Part model, mm, in its own coordinate system. A direction names the side the tool comes from. Round coordinates to 2 decimals unless told otherwise and drop trailing zeros. Order: outer loops, then holes, each group sorted by start corner. A loop starts at its lowest first (then second) coordinate and runs counter-clockwise, first axis right, second up. Notation, with made-up numbers: M 21,71 L 34,71 A14 cw 34,77 Z; hole C -26,39 d4. An arc over 180 degrees is marked long. Write each question's results on one line, items separated by ' | '. Start each with the question number.
1. Band-saw the part on C-C, the plane x = 40. List the corners of the cut face in (y, z).
2. Two-plate mould, pull along X, no slides. Class faces 3 (the face through (69.89, -30.02, 7.46)), 4 (the face through (41.068, -25.451, 7.465)), 5 (the face through (84.52, -17.57, 7.46)): +X half, -X half, draft (parallel to the pull), parting line (faces both ways), or undercut.
3. Band-saw the part on D-D, the plane z = 8.45. Give the number of separate pieces and of enclosed holes in the cut face, then the cut area to 3 significant figures.
4. Probe L1, parallel to Y at x = 60, z = 5.9; L2, parallel to Y at x = 49.5, z = 8.9; L3, parallel to X at y = -24.5, z = 7.8. List the from-to ranges inside material, lowest first. Write a range as [from, to].
5. Drop flat-ended pins along their axis: pin 1 Ø3.5 at (x, y) = (59.85, -25.73) entering from -Z; pin 2 Ø2 at (y, z) = (-3.5, 9) entering from -X; pin 3 Ø1 at (y, z) = (-14, 9.5) entering from -X. Give the stop position or say it passes through.
6. Band-saw the part on B-B, the plane x = 62.5. List the corners of the cut face in (y, z), then the cut area to 3 significant figures.
7. Which spindle directions (+Z, -Z, +X, -X, +Y, -Y) get a long thin tool onto all of the face, cutting with end or side? Do faces 1 (the face through (45, 0, 7)), 2 (the face through (93.45, -26.96, 7.54)). Say none if no direction does.
8. Band-saw the part on A-A, the plane y = 0. List the corners of the cut face in (x, z), then the cut area to 3 significant figures.
```python
from build123d import *

# Parameters (mm, degrees)
EXTRUDE_1_DEPTH     = 15
FILLET_1_R          = 5
FILLET_2_R          = 5
FILLET_3_R          = 5
FILLET_4_R          = 5
FILLET_5_R          = 5
FILLET_6_R          = 5
FILLET_7_R          = 5
FILLET_8_R          = 5
FILLET_9_R          = 5
FILLET_10_R         = 5
FILLET_11_R         = 5
FILLET_12_R         = 5
FILLET_13_R         = 5
FILLET_14_R         = 5
FILLET_15_R         = 5
FILLET_16_R         = 5
SKETCH_5_R          = 1.5
CUT_EXTRUDE_1_DEPTH = 15
CUT_EXTRUDE_START   = -15
SKETCH_6_R          = 1.5
CUT_EXTRUDE_5_DEPTH = 15
EXTRUDE_2_DEPTH     = 15
FILLET_17_R         = 5
FILLET_18_R         = 5
FILLET_19_R         = 5
FILLET_20_R         = 5
SKETCH_8_W          = 96.520141499
SKETCH_8_H          = 72.316132992
CUT_EXTRUDE_6_DEPTH = 5
SKETCH_9_W          = 91.216327174
SKETCH_9_H          = 79.967676963
CUT_EXTRUDE_7_DEPTH = 5


with BuildPart() as part:
    # 草图3 → 凸台-拉伸1 (new body)
    with BuildSketch(Plane.XY):
        with BuildLine():
            Line((101.99145665, -27.727634828), (114.18506552, -15.283623844))
            ThreePointArc((114.18506552, -15.283623844), (110, 0), (114.18506552, 15.283623844))
            Line((114.18506552, 15.283623844), (101.99145665, 27.727634828))
            Line((101.99145665, 27.727634828), (48.171786379, 31.57189699))
            Line((48.171786379, 31.57189699), (32.743622368, 18.278544642))
            ThreePointArc((32.743622368, 18.278544642), (37.5, 0), (32.743622368, -18.278544642))
            Line((32.743622368, -18.278544642), (48.171786379, -31.57189699))
            Line((48.171786379, -31.57189699), (101.99145665, -27.727634828))
        make_face()
        with BuildLine():
            ThreePointArc((42.839131819, -13.777110909), (45, 0), (42.839131819, 13.777110909))
            Line((42.839131819, 13.777110909), (51.574083604, 21.303398011))
            Line((51.574083604, 21.303398011), (97.500283316, 18.022955175))
            Line((97.500283316, 18.022955175), (106.212331228, 9.132000819))
            ThreePointArc((106.212331228, 9.132000819), (105, 0), (106.212331228, -9.132000819))
            Line((106.212331228, -9.132000819), (97.500283316, -18.022955175))
            Line((97.500283316, -18.022955175), (51.574083604, -21.303398011))
            Line((51.574083604, -21.303398011), (42.839131819, -13.777110909))
        make_face(mode=Mode.SUBTRACT)
    extrude(amount=EXTRUDE_1_DEPTH)

    # 圆角1
    fillet_1_edges = [part.edges().sort_by_distance(p)[0] for p in [
        (101.99145665, 27.727634828, 7.5),
    ]]
    fillet(fillet_1_edges, radius=FILLET_1_R)

    # 圆角2
    fillet_2_edges = [part.edges().sort_by_distance(p)[0] for p in [
        (114.18506552, 15.283623844, 7.5),
    ]]
    fillet(fillet_2_edges, radius=FILLET_2_R)

    # 圆角3
    fillet_3_edges = [part.edges().sort_by_distance(p)[0] for p in [
        (114.18506552, -15.283623844, 7.5),
    ]]
    fillet(fillet_3_edges, radius=FILLET_3_R)

    # 圆角4
    fillet_4_edges = [part.edges().sort_by_distance(p)[0] for p in [
        (101.99145665, -27.727634828, 7.5),
    ]]
    fillet(fillet_4_edges, radius=FILLET_4_R)

    # 圆角5
    fillet_5_edges = [part.edges().sort_by_distance(p)[0] for p in [
        (48.171786379, -31.57189699, 7.5),
    ]]
    fillet(fillet_5_edges, radius=FILLET_5_R)

    # 圆角6
    fillet_6_edges = [part.edges().sort_by_distance(p)[0] for p in [
        (48.171786379, 31.57189699, 7.5),
    ]]
    fillet(fillet_6_edges, radius=FILLET_6_R)

    # 圆角7
    fillet_7_edges = [part.edges().sort_by_distance(p)[0] for p in [
        (32.743622368, -18.278544642, 7.5),
    ]]
    fillet(fillet_7_edges, radius=FILLET_7_R)

    # 圆角8
    fillet_8_edges = [part.edges().sort_by_distance(p)[0] for p in [
        (32.743622368, 18.278544642, 7.5),
    ]]
    fillet(fillet_8_edges, radius=FILLET_8_R)

    # 圆角9
    fillet_9_edges = [part.edges().sort_by_distance(p)[0] for p in [
        (97.500283316, -18.022955175, 7.5),
    ]]
    fillet(fillet_9_edges, radius=FILLET_9_R)

    # 圆角10
    fillet_10_edges = [part.edges().sort_by_distance(p)[0] for p in [
        (106.212331228, -9.132000819, 7.5),
    ]]
    fillet(fillet_10_edges, radius=FILLET_10_R)

    # 圆角11
    fillet_11_edges = [part.edges().sort_by_distance(p)[0] for p in [
        (106.212331228, 9.132000819, 7.5),
    ]]
    fillet(fillet_11_edges, radius=FILLET_11_R)

    # 圆角12
    fillet_12_edges = [part.edges().sort_by_distance(p)[0] for p in [
        (97.500283316, 18.022955175, 7.5),
    ]]
    fillet(fillet_12_edges, radius=FILLET_12_R)

    # 圆角13
    fillet_13_edges = [part.edges().sort_by_distance(p)[0] for p in [
        (51.574083604, -21.303398011, 7.5),
    ]]
    fillet(fillet_13_edges, radius=FILLET_13_R)

    # 圆角14
    fillet_14_edges = [part.edges().sort_by_distance(p)[0] for p in [
        (42.839131819, -13.777110909, 7.5),
    ]]
    fillet(fillet_14_edges, radius=FILLET_14_R)

    # 圆角15
    fillet_15_edges = [part.edges().sort_by_distance(p)[0] for p in [
        (42.839131819, 13.777110909, 7.5),
    ]]
    fillet(fillet_15_edges, radius=FILLET_15_R)

    # 圆角16
    fillet_16_edges = [part.edges().sort_by_distance(p)[0] for p in [
        (51.574083604, 21.303398011, 7.5),
    ]]
    fillet(fillet_16_edges, radius=FILLET_16_R)

    # 草图5 → 切除-拉伸1 (cut)
    with BuildSketch(Plane(origin=(0, 0, 0), x_dir=(-1, 0, 0), z_dir=(0, 0, -1))):
        with Locations((-36.9551813, 15.307337295)):
            Circle(SKETCH_5_R)
        with Locations((-40, 0)):
            Circle(SKETCH_5_R)
        with Locations((-36.9551813, -15.307337295)):
            Circle(SKETCH_5_R)
        with Locations((-49.872934992, -26.437647501)):
            Circle(SKETCH_5_R)
        with Locations((-49.872934992, 26.437647501)):
            Circle(SKETCH_5_R)
        with Locations((-99.745869983, 22.875295001)):
            Circle(SKETCH_5_R)
        with Locations((-99.745869983, -22.875295001)):
            Circle(SKETCH_5_R)
        with Locations((-109.973915193, 12.437211552)):
            Circle(SKETCH_5_R)
        with Locations((-107.5, 0)):
            Circle(SKETCH_5_R)
        with Locations((-109.973915193, -12.437211552)):
            Circle(SKETCH_5_R)
        with Locations((-59.84752199, 25.725177001)):
            Circle(SKETCH_5_R)
        with Locations((-69.822108988, 25.012706501)):
            Circle(SKETCH_5_R)
        with Locations((-79.796695986, 24.300236001)):
            Circle(SKETCH_5_R)
        with Locations((-89.771282985, 23.587765501)):
            Circle(SKETCH_5_R)
        with Locations((-89.771282985, -23.587765501)):
            Circle(SKETCH_5_R)
        with Locations((-79.796695986, -24.300236001)):
            Circle(SKETCH_5_R)
        with Locations((-69.822108988, -25.012706501)):
            Circle(SKETCH_5_R)
        with Locations((-59.84752199, -25.725177001)):
            Circle(SKETCH_5_R)
    extrude(amount=-CUT_EXTRUDE_1_DEPTH, mode=Mode.SUBTRACT)

    # 草图6 → 切除-拉伸5 (cut)
    # profile 1 of 5: a face of its own
    with BuildSketch(Plane.XY.offset(15).offset(CUT_EXTRUDE_START)):
        with BuildLine():
            ThreePointArc((103.31715251, 26.374715112), (101.845820167, 27.412938577), (100.102105233, 27.8625885))
            Line((100.102105233, 27.8625885), (100.102105233, 24.332379915))
            ThreePointArc((100.102105233, 24.332379915), (100.925775249, 23.801482651), (101.245869983, 22.875295001))
            ThreePointArc((101.245869983, 22.875295001), (100.925775249, 21.949107351), (100.102105233, 21.418210087))
            Line((100.102105233, 21.418210087), (100.102105233, 15.367703489))
            Line((100.102105233, 15.367703489), (104.297377986, 11.086278624))
            ThreePointArc((104.297377986, 11.086278624), (105.514152308, 9.027175008), (105.635333526, 6.638501199))
            ThreePointArc((105.635333526, 6.638501199), (105, 0), (105.635333526, -6.638501199))
            ThreePointArc((105.635333526, -6.638501199), (105.514152308, -9.027175008), (104.297377986, -11.086278624))
            Line((104.297377986, -11.086278624), (100.102105233, -15.367703489))
            Line((100.102105233, -15.367703489), (100.102105233, -21.418210087))
            ThreePointArc((100.102105233, -21.418210087), (100.925775249, -21.949107351), (101.245869983, -22.875295001))
            ThreePointArc((101.245869983, -22.875295001), (100.925775249, -23.801482651), (100.102105233, -24.332379915))
            Line((100.102105233, -24.332379915), (100.102105233, -27.8625885))
            ThreePointArc((100.102105233, -27.8625885), (101.845820167, -27.412938577), (103.31715251, -26.374715112))
            Line((103.31715251, -26.374715112), (111.655402821, -17.865234485))
            ThreePointArc((111.655402821, -17.865234485), (113.00675492, -15.241981218), (112.643531681, -12.313555178))
            ThreePointArc((112.643531681, -12.313555178), (110, 0), (112.643531681, 12.313555178))
            ThreePointArc((112.643531681, 12.313555178), (113.00675492, 15.241981218), (111.655402821, 17.865234485))
            Line((111.655402821, 17.865234485), (103.31715251, 26.374715112))
        make_face()
        with Locations((109.973915193, -12.437211552)):
            Circle(SKETCH_6_R, mode=Mode.SUBTRACT)
        with Locations((107.5, 0)):
            Circle(SKETCH_6_R, mode=Mode.SUBTRACT)
        with Locations((109.973915193, 12.437211552)):
            Circle(SKETCH_6_R, mode=Mode.SUBTRACT)
    # profile 2 of 5: a face of its own
    with BuildSketch(Plane.XY.offset(15).offset(CUT_EXTRUDE_START)):
        with BuildLine():
            Line((100.102105233, -21.418210087), (100.102105233, -15.367703489))
            Line((100.102105233, -15.367703489), (98.825979176, -16.670035459))
            ThreePointArc((98.825979176, -16.670035459), (97.354646834, -17.708258924), (95.610931899, -18.157908847))
            Line((95.610931899, -18.157908847), (94.758576484, -18.218791377))
            Line((94.758576484, -18.218791377), (94.758576484, -23.231530251))
            Line((94.758576484, -23.231530251), (98.249681933, -22.982165576))
            ThreePointArc((98.249681933, -22.982165576), (98.778211836, -21.729154647), (100.102105233, -21.418210087))
        make_face()
    # profile 3 of 5: a face of its own
    with BuildSketch(Plane.XY.offset(15).offset(CUT_EXTRUDE_START)):
        with BuildLine():
            Line((94.758576484, -28.244269125), (100.102105233, -27.8625885))
            Line((100.102105233, -27.8625885), (100.102105233, -24.332379915))
            ThreePointArc((100.102105233, -24.332379915), (98.862330065, -24.087465457), (98.249681933, -22.982165576))
            Line((98.249681933, -22.982165576), (94.758576484, -23.231530251))
            Line((94.758576484, -23.231530251), (94.758576484, -28.244269125))
        make_face()
    # profile 4 of 5: a face of its own
    with BuildSketch(Plane.XY.offset(15).offset(CUT_EXTRUDE_START)):
        with BuildLine():
            Line((100.102105233, 15.367703489), (100.102105233, 21.418210087))
            ThreePointArc((100.102105233, 21.418210087), (98.778211836, 21.729154647), (98.249681933, 22.982165576))
            Line((98.249681933, 22.982165576), (94.758576484, 23.231530251))
            Line((94.758576484, 23.231530251), (94.758576484, 18.218791377))
            Line((94.758576484, 18.218791377), (95.610931899, 18.157908847))
            ThreePointArc((95.610931899, 18.157908847), (97.354646834, 17.708258924), (98.825979176, 16.670035459))
            Line((98.825979176, 16.670035459), (100.102105233, 15.367703489))
        make_face()
    # profile 5 of 5: a face of its own
    with BuildSketch(Plane.XY.offset(15).offset(CUT_EXTRUDE_START)):
        with BuildLine():
            Line((100.102105233, 24.332379915), (100.102105233, 27.8625885))
            Line((100.102105233, 27.8625885), (94.758576484, 28.244269125))
            Line((94.758576484, 28.244269125), (94.758576484, 23.231530251))
            Line((94.758576484, 23.231530251), (98.249681933, 22.982165576))
            ThreePointArc((98.249681933, 22.982165576), (98.862330065, 24.087465457), (100.102105233, 24.332379915))
        make_face()
    extrude(amount=CUT_EXTRUDE_5_DEPTH, mode=Mode.SUBTRACT)

    # 草图7 → 凸台-拉伸2 (add)
    with BuildSketch(Plane.XY.offset(15)):
        Polygon((94.758576484, -18.218791377), (94.758576484, 18.218791377), (85.826771952, 18.856777415), (85.826771952, -18.856777415), align=None)
    extrude(amount=-EXTRUDE_2_DEPTH)

    # 圆角17
    fillet_17_edges = [part.edges().sort_by_distance(p)[0] for p in [
        (94.758576484, 28.244269125, 7.5),
    ]]
    fillet(fillet_17_edges, radius=FILLET_17_R)

    # 圆角18
    fillet_18_edges = [part.edges().sort_by_distance(p)[0] for p in [
        (94.758576484, -28.244269125, 7.5),
    ]]
    fillet(fillet_18_edges, radius=FILLET_18_R)

    # 圆角19
    fillet_19_edges = [part.edges().sort_by_distance(p)[0] for p in [
        (85.826771952, 18.856777415, 7.5),
    ]]
    fillet(fillet_19_edges, radius=FILLET_19_R)

    # 圆角20
    fillet_20_edges = [part.edges().sort_by_distance(p)[0] for p in [
        (85.826771952, -18.856777415, 7.5),
    ]]
    fillet(fillet_20_edges, radius=FILLET_20_R)

    # 草图8 → 切除-拉伸6 (cut)
    with BuildSketch(Plane(origin=(0, 0, 0), x_dir=(-1, 0, 0), z_dir=(0, 0, -1))):
        with Locations((-67.250576804, -3.787424314)):
            Rectangle(SKETCH_8_W, SKETCH_8_H)
    extrude(amount=-CUT_EXTRUDE_6_DEPTH, mode=Mode.SUBTRACT)

    # 草图9 → 切除-拉伸7 (cut)
    with BuildSketch(Plane.XY.offset(15)):
        with Locations((64.504220749, 0.715823196)):
            Rectangle(SKETCH_9_W, SKETCH_9_H)
    extrude(amount=-CUT_EXTRUDE_7_DEPTH, mode=Mode.SUBTRACT)


solid = part.part
```
Solution:
1) outline: M -24.53,5 L -1.5,5 L -1.5,10 L -24.53,10 Z; M 1.5,5 L 24.53,5 L 24.53,10 L 1.5,10 Z
2) face 3: +X half | face 4: -X half | face 5: undercut
3) separate pieces: 1 | enclosed holes: 14 | area: 1,700 mm^2
4) L1: [-30.73, -27.22], [-24.23, -20.7], [20.7, 24.23], [27.22, 30.73] | L2: [-31.42, -27.89], [-24.98, -19.52], [19.52, 24.98], [27.89, 31.42] | L3: [39.96, 58.98], [60.71, 68.41], [71.23, 78.31], [81.28, 88.58], [90.96, 94.67]
5) pin 1: z = 5 | pin 2: x = 37.23 | pin 3: x = 34.58
6) outline: M -30.55,5 L -20.52,5 L -20.52,10 L -30.55,10 Z; M 20.52,5 L 30.55,5 L 30.55,10 L 20.52,10 Z | area: 100 mm^2
7) face 1: +Z, -Z | face 2: +Z, -Z, +X, -Y
8) outline: M 37.5,5 L 38.5,5 L 38.5,10 L 37.5,10 Z; M 41.5,5 L 45,5 L 45,10 L 41.5,10 Z; M 85.83,5 L 94.76,5 L 94.76,10 L 85.83,10 Z | area: 67.2 mm^2
